Verification items for this drawing (mm, ordinates from the low corner). A direction names the side the tool comes from. Round coordinates to 2 decimals unless told otherwise and drop trailing zeros. Write each loop counter-clockwise with the first axis right and the second up, starting at its lowest first coordinate (ties: lowest second). Pieces come first, ordered by that corner, then holes. Notation, with made-up numbers: (-5, 52.25) -> (22, 52.25) arc R8 cw to (22, 56.25) -> close; hole circle Ø6 at (44.5, -17.5). An arc over 180 degrees is marked (long way). One line per item, written item: value.
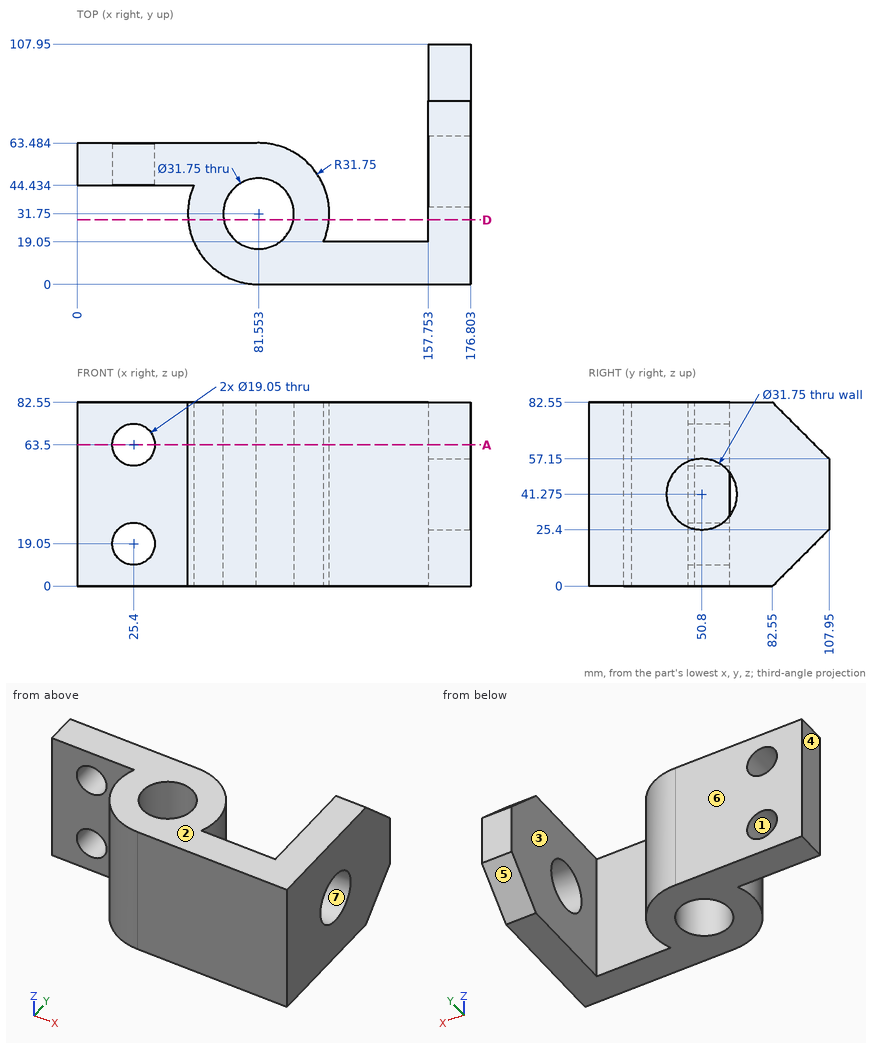
Item 1: Sectioned sample at D-D (y = 29). Enter the section's corners in (x, z).
Result set:
outline: (49.92, 0) -> (65.92, 0) -> (65.92, 82.55) -> (49.92, 82.55) -> close; (97.19, 0) -> (113.18, 0) -> (113.18, 82.55) -> (97.19, 82.55) -> close; (157.75, 0) -> (176.8, 0) -> (176.8, 82.55) -> (157.75, 82.55) -> close
Item 2: Release check for a two-part mould opening along X. For the marked faces 1, 2, 3 and 4 record: pulls with the +X half, pulls with the -X half, needs draft (parallel to the pull), parting line crosses it, or undercut.
Result set:
face 1: undercut
face 2: needs draft
face 3: undercut
face 4: pulls with the -X half
Item 3: Tool access check on the marked faces 5, 6 and 7. Record the directions out of +Z, -Z, +X, -X, +Y, -Y that give a thin tool (end or side, any length) a straight path to the whole face; none if there is none.
Result set:
face 5: -Z, +X, -X, +Y
face 6: +Z, -Z, -X, +Y
face 7: +X
Item 4: Material ranges on line 1 along X through (y, z) = (31, 27) (1 decimal); line 2 along X through (y, z) = (27.5, 69.5); line 3 along Y through (x, z) = (125.5, 60.5), recorded low to high.
Result set:
line 1: 49.8 to 65.7, 97.4 to 113.3, 157.8 to 176.8
line 2: 50.09 to 66.26, 96.85 to 113.02, 157.75 to 176.8
line 3: 0 to 19.05
Item 5: Depth check by flat-ended pin: pin 1 (5 mm diameter, centred on x = 23, z = 70, fed in from -Y); pin 2 (12 mm diameter, centred on x = 57.5, z = 39, fed in from -Y); pin 3 (22 mm diameter, centred on x = 25.4, z = 63.5, fed in from +Y); pin 4 (4 mm diameter, centred on y = 87.5, z = 63.5, fed in from -X). Enter the tip coordinate at first touch or a pass-through.
Result set:
pin 1: through
pin 2: y = 5.63
pin 3: y = 63.48
pin 4: x = 157.75
Item 6: Sectioned sample at A-A (z = 63.5). State how many separate pieces and enclosed holes the cut face has, then the cut area to 3 significant figures.
Result set:
separate pieces: 2
enclosed holes: 1
area: 6,150 mm^2
